Model file for the job. Use its own axes, mm. Coordinates: 2 decimals unless noted, no trailing zeros. Order: outer loops, then holes, each group sorted by start corner. A loop starts at its lowest first (then second) coordinate and runs counter-clockwise, first axis right, second up. Notation, with made-up numbers: (49.5, 31.5) -> (78.5, 31.5) arc R16 cw to (78.5, 50.5) -> close; hole circle Ø7 at (-9, -33.75). An arc over 180 degrees is marked (long way). Write item = value, one per line. Start each with the question number.
Q1. Wall check: line 1 (X direction, y = 12.5, z = 4); line 2 (Z direction, x = 7, y = 25); line 3 (Y direction, x = 12, z = 4.75). Give the ranges that are in metal, low to high. Write a range as from..to.
Q2. Cut at D-D, the plane x = -22.5. List the corners of the cut face in (y, z), plus the area to 3 significant figures.
Q3. Cut at A-A, the plane x = 0. List the corners of the cut face in (y, z).
Q4. Cut at B-B, the plane y = 12.5. Give the number of separate pieces and of enclosed holes in the cut face, plus the area to 3 significant figures.
Q5. Flat gauge pins, fed straight in: pin 1 (8.5 mm diameter, centred on x = 7, y = 12.5, fed in from -Z); pin 2 (2 mm diameter, centred on x = 13, z = 7.901, fed in from +Y); pin 3 (1.2 mm diameter, centred on x = -7, z = -2.5, fed in from +Y); pin 4 (1.5 mm diameter, centred on x = 0, y = 2.5, fed in from +Z). Where does each tip first touch, or does it go through?
Q6. Cut at C-C, the plane y = -16. List the corners of the cut face in (x, z), plus the area to 3 significant figures.
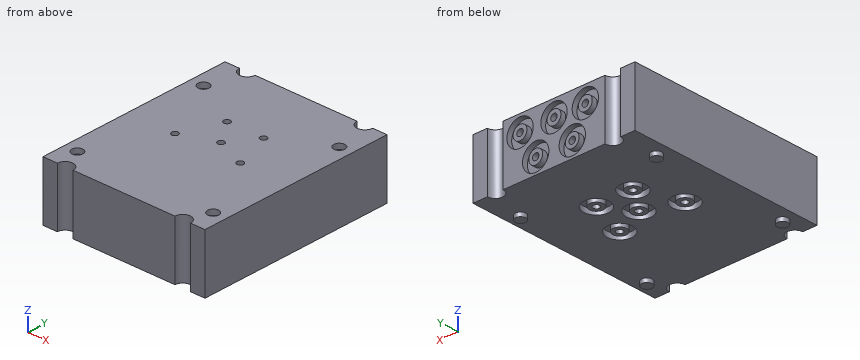
from build123d import *

# Parameters (mm, degrees)
F0_W      = 62
F0_H      = 75
F1_DEPTH  = 14
F2_W      = 62
F2_H      = 75
F3_DEPTH  = 8
F4_R      = 1.25
F5_DEPTH  = 38
F6_R      = 4.85
F6_R_2    = 2.65
F7_DEPTH  = 2
F8_R      = 2.1
F9_DEPTH  = 2
F10_R     = 1.25
F11_DEPTH = 35.5
F12_R     = 5.05
F12_R_2   = 2.65
F13_DEPTH = 2
F14_DEPTH = 27.2
F15_DEPTH = 18.2
F17_DEPTH = 25
F18_R     = 2
F19_DEPTH = 1.5


with BuildPart() as f1:
    # F0 (on Top) → F1 (new body)
    with BuildSketch(Plane.XY):
        Rectangle(F0_W, F0_H)
    extrude(amount=F1_DEPTH)

    # F2 (on face) → F3 (join)
    with BuildSketch(Plane(origin=(0, 0, 0), x_dir=(1, 0, 0), z_dir=(0, 0, -1))):
        Rectangle(F2_W, F2_H)
    extrude(amount=F3_DEPTH)

    # F4 (on face) → F5 (cut)
    with BuildSketch(Plane(origin=(0, 0, -8), x_dir=(1, 0, 0), z_dir=(0, 0, -1))):
        with Locations((-13, 2.5)):
            Circle(F4_R)
        with Locations((-7, -12.5)):
            Circle(F4_R)
        with Locations((0, -2.5)):
            Circle(F4_R)
        with Locations((7, -12.5)):
            Circle(F4_R)
        with Locations((12, 2.5)):
            Circle(F4_R)
    extrude(amount=-F5_DEPTH, mode=Mode.SUBTRACT)

    # F6 (on face) → F7 (cut)
    with BuildSketch(Plane(origin=(0, 0, -8), x_dir=(1, 0, 0), z_dir=(0, 0, -1))):
        with Locations((-7, -12.5)):
            Circle(F6_R)
        with Locations((-7, -12.5)):
            Circle(F6_R_2, mode=Mode.SUBTRACT)
        with Locations((-13, 2.5)):
            Circle(F6_R)
        with Locations((-13, 2.5)):
            Circle(F6_R_2, mode=Mode.SUBTRACT)
        with Locations((0, -2.5)):
            Circle(F6_R)
        with Locations((0, -2.5)):
            Circle(F6_R_2, mode=Mode.SUBTRACT)
        with Locations((12, 2.5)):
            Circle(F6_R)
        with Locations((12, 2.5)):
            Circle(F6_R_2, mode=Mode.SUBTRACT)
        with Locations((7, -12.5)):
            Circle(F6_R)
        with Locations((7, -12.5)):
            Circle(F6_R_2, mode=Mode.SUBTRACT)
    extrude(amount=-F7_DEPTH, mode=Mode.SUBTRACT)

    # F8 (on face) → F9 (cut)
    with BuildSketch(Plane.XY.offset(14)):
        with Locations((-26, 23.2629562748)):
            Circle(F8_R)
        with Locations((26, 23.2629562748)):
            Circle(F8_R)
        with Locations((26, -28.7370437252)):
            Circle(F8_R)
        with Locations((-26, -28.7370437252)):
            Circle(F8_R)
    extrude(amount=-F9_DEPTH, mode=Mode.SUBTRACT)

    # F10 (on face) → F11 (cut)
    with BuildSketch(Plane(origin=(0, 37.5, 0), x_dir=(-1, 0, 0), z_dir=(0, 1, 0))):
        with Locations((12, 7.901)):
            Circle(F10_R)
        with Locations((-13, 7.901)):
            Circle(F10_R)
    extrude(amount=-F11_DEPTH, mode=Mode.SUBTRACT)

    # F12 (on face) → F13 (cut)
    with BuildSketch(Plane(origin=(0, 37.5, 0), x_dir=(-1, 0, 0), z_dir=(0, 1, 0))):
        with Locations((-13, 7.901)):
            Circle(F12_R)
        with Locations((-13, 7.901)):
            Circle(F12_R_2, mode=Mode.SUBTRACT)
        with Locations((-7, -2.099)):
            Circle(F12_R)
        with Locations((-7, -2.099)):
            Circle(F12_R_2, mode=Mode.SUBTRACT)
        with Locations((0, 7.901)):
            Circle(F12_R)
        with Locations((0, 7.901)):
            Circle(F12_R_2, mode=Mode.SUBTRACT)
        with Locations((7, -2.099)):
            Circle(F12_R)
        with Locations((7, -2.099)):
            Circle(F12_R_2, mode=Mode.SUBTRACT)
        with Locations((12, 7.901)):
            Circle(F12_R)
        with Locations((12, 7.901)):
            Circle(F12_R_2, mode=Mode.SUBTRACT)
    extrude(amount=-F13_DEPTH, mode=Mode.SUBTRACT)

    # F10 (on face) → F14 (cut)
    with BuildSketch(Plane(origin=(0, 37.5, 0), x_dir=(-1, 0, 0), z_dir=(0, 1, 0))):
        with Locations((0, 7.901)):
            Circle(F10_R)
    extrude(amount=-F14_DEPTH, mode=Mode.SUBTRACT)

    # F10 (on face) → F15 (cut)
    with BuildSketch(Plane(origin=(0, 37.5, 0), x_dir=(-1, 0, 0), z_dir=(0, 1, 0))):
        with Locations((7, -2.099)):
            Circle(F10_R)
        with Locations((-7, -2.099)):
            Circle(F10_R)
    extrude(amount=-F15_DEPTH, mode=Mode.SUBTRACT)

    # F16 (on face) → F17 (cut)
    with BuildSketch(Plane(origin=(0, 0, -8), x_dir=(1, 0, 0), z_dir=(0, 0, -1))):
        with BuildLine():
            ThreePointArc((-25.5, 37.5), (-22.5, 34.5), (-19.5, 37.5))
            Line((-19.5, 37.5), (-25.5, 37.5))
        make_face()
        with BuildLine():
            Line((25.5, 37.5), (19.5, 37.5))
            ThreePointArc((19.5, 37.5), (22.5, 34.5), (25.5, 37.5))
        make_face()
        with BuildLine():
            ThreePointArc((-19.5, -37.5), (-22.5, -34.5), (-25.5, -37.5))
            Line((-25.5, -37.5), (-19.5, -37.5))
        make_face()
        with BuildLine():
            Line((19.5, -37.5), (25.5, -37.5))
            ThreePointArc((25.5, -37.5), (22.5, -34.5), (19.5, -37.5))
        make_face()
    extrude(amount=-F17_DEPTH, mode=Mode.SUBTRACT)

    # F18 (on face) → F19 (join)
    with BuildSketch(Plane(origin=(0, 0, -8), x_dir=(1, 0, 0), z_dir=(0, 0, -1))):
        with Locations((-26, 28.7370437252)):
            Circle(F18_R)
        with Locations((26, 28.7370437252)):
            Circle(F18_R)
        with Locations((26, -23.2629562748)):
            Circle(F18_R)
        with Locations((-26, -23.2629562748)):
            Circle(F18_R)
    extrude(amount=F19_DEPTH)


solid = f1.part
Here are the results:
q1.line_1 = -31..-8.25, -5.75..5.75, 8.25..31
q1.line_2 = -8..-3.35, -0.85..14
q1.line_3 = -37.5..-3.75, -1.25..35.5
q2.outline = (-34.5, -8) -> (34.5, -8) -> (34.5, 14) -> (-34.5, 14) -> close
q2.area = 1,520 mm²
q3.outline = (-37.5, -8) -> (-2.35, -8) -> (-2.35, -6) -> (-0.15, -6) -> (-0.15, -8) -> (1.25, -8) -> (1.25, 14) -> (-37.5, 14) -> close; (3.75, -8) -> (5.15, -8) -> (5.15, -6) -> (7.35, -6) -> (7.35, -8) -> (37.5, -8) -> (37.5, 2.85) -> (35.5, 2.85) -> (35.5, 5.25) -> (37.5, 5.25) -> (37.5, 6.65) -> (10.3, 6.65) -> (10.3, 9.15) -> (37.5, 9.15) -> (37.5, 10.55) -> (35.5, 10.55) -> (35.5, 12.95) -> (37.5, 12.95) -> (37.5, 14) -> (3.75, 14) -> close
q4.separate_pieces = 3
q4.enclosed_holes = 3
q4.area = 1,220 mm²
q5.pin_1 = -8
q5.pin_2 = 2
q5.pin_3 = 19.3
q5.pin_4 = through
q6.outline = (-31, -8) -> (31, -8) -> (31, 14) -> (-31, 14) -> close
q6.area = 1,360 mm²
